Input: part model. Units: mm. Frame: model coordinates. A direction names the side the tool comes from. Coordinates: 2 decimals unless noted, no trailing zeros. Order: outer loops, then holes, each group sorted by start corner. A loop starts at its lowest first (then second) coordinate and runs counter-clockwise, first axis right, second up. Notation, with made-up numbers: (-13.75, -18) - (-7.75, -18) arc R20 ccw to (-7.75, -12) - close; hole circle Ø11 at (-39, 3.25). An arc over 180 degrees is marked (long way). Answer as CSV lines item,"result". Start each with the question number.
Item 1: First-contact query: pin 1 (8 mm diameter, centred on y = 14, z = 7.5, fed in from +X); pin 2 (8 mm diameter, centred on x = 8, z = -5, fed in from +Y); pin 3 (6 mm diameter, centred on x = -14.72, y = -8.5, fed in from +Z); pin 4 (6 mm diameter, centred on x = 0, y = -17, fed in from -Z). Flat tips, straight axial feed; report the tip coordinate or a pass-through.
Item 2: Draft query along X for faces 3 (the cylindrical face through (14.18, -10.94, 5.07)), 4 (the flat face through (4, -4, 10)), 5 (the cylindrical face through (-11.923, -3.755, -7.395)). Return one class per face: +X half, -X half, draft (parallel to the pull), parting line (faces both ways), or undercut.
Item 3: Section D-D (z = -5). Output: boundary loops of the cut face in (x, y).
Item 4: Section B-B (y = -8.5). Output: boundary loops of the cut face in (x, z).
Item 5: Section C-C (y = 0). Output: boundary loops of the cut face in (x, z), and give its area (3 significant figures).
Item 6: Access query for faces 1 (the flat face through (9, -9, 0)), 2 (the cylindrical face through (14.18, 6.06, 5.07)). Directions: +Z, -Z, +X, -X, +Y, -Y. A direction counts if a zero-diameter tool reaches every point of the face in a straight line with its end or side. Return the directions, or none.
Item 7: Section A-A (x = 0). Output: boundary loops of the cut face in (y, z), and give its area (3 significant figures).
Item 8: Material intervals for line 1 along Y through (x, z) = (0, 3.25); line 2 along X through (y, z) = (8.5, 3.5); line 3 along Y through (x, z) = (-2, 5), sorted ascending.
Autodesk Inventor part; units mm, degrees
ref_plane "YZ Plane" through (0, 0, 0) normal (1, 0, 0) x (0, 1, 0)
ref_plane "XZ Plane" through (0, 0, 0) normal (0, 1, 0) x (-1, 0, 0)
ref_plane "XY Plane" through (0, 0, 0) normal (0, 0, 1) x (1, 0, 0)
sketch "Szkic1" plane through (0, 0, 0) normal (0, 0, 1) x (1, 0, 0)
  circle A0 centre (0, 0) radius 21
  dimension "d0" = 42
extrude "Wyciągnięcie proste1" add sketch "Szkic1" along normal blind 10
sketch "Szkic2" plane through (0, 0, 10) normal (0, 0, 1) x (1, 0, 0)
  circle A0 centre (0, 0) radius 17
  circle A1 centre (0, 17) radius 2.5
  circle A2 centre (14.7224, 8.5) radius 2.5
  circle A3 centre (14.7224, -8.5) radius 2.5
  circle A4 centre (0, -17) radius 2.5
  circle A5 centre (-14.7224, -8.5) radius 2.5
  circle A6 centre (-14.7224, 8.5) radius 2.5
  dimension "d3" = 34
  dimension "d4" = 5
  dimension "d7" = 360
extrude "Wyciągnięcie proste2" cut sketch "Szkic2" against normal up to next contours A2 A0 | A0 A2 | A3 A0 | A0 A3 | A1 A0 | A0 A1 | A4 A0 | A0 A4 | A6 A0 | A0 A6 | A5 A0 | A0 A5
sketch "Szkic3" plane through (0, 0, 10) normal (0, 0, 1) x (1, 0, 0)
  circle A0 centre (0, 0) radius 5
  dimension "d11" = 10
extrude "Wyciągnięcie proste3" cut sketch "Szkic3" against normal up to next
sketch "Szkic4" plane through (0, 0, 0) normal (0, 0, -1) x (-1, 0, 0)
  circle A0 centre (0, 0) radius 5
  circle A1 centre (0, 0) radius 12.5
  dimension "d14" = 25
extrude "Wyciągnięcie proste4" add sketch "Szkic4" along normal blind 15
thread "Gwint1"
properties part number "Nakrętka trapezowa kołnierzowa JFRM-2525TR10x3"
Determined:
1,pin 1,"stops at x = 18.47"
1,pin 2,"stops at y = 11.84"
1,pin 3,"stops at z = 10"
1,pin 4,"stops at z = 0"
2,face 3,"undercut"
2,face 4,"draft"
2,face 5,"parting line"
3,outline,"circle Ø25 at (0, 0); hole circle Ø10 at (0, 0)"
4,outline,"(-19.2, 0) - (-17.22, 0) - (-17.22, 10) - (-19.2, 10) - close; (-12.22, 0) - (-9.17, 0) - (-9.17, -15) - (9.17, -15) - (9.17, 0) - (12.22, 0) - (12.22, 10) - (-12.22, 10) - close; (17.22, 0) - (19.2, 0) - (19.2, 10) - (17.22, 10) - close"
5,outline,"(-21, 0) - (-12.5, 0) - (-12.5, -15) - (-5, -15) - (-5, 10) - (-21, 10) - close; (5, -15) - (12.5, -15) - (12.5, 0) - (21, 0) - (21, 10) - (5, 10) - close"
5,area,"545 mm^2"
6,face 1,"-Z"
6,face 2,"+Z, -Z"
7,outline,"(-21, 0) - (-19.5, 0) - (-19.5, 10) - (-21, 10) - close; (-14.5, 0) - (-12.5, 0) - (-12.5, -15) - (-5, -15) - (-5, 10) - (-14.5, 10) - close; (5, -15) - (12.5, -15) - (12.5, 0) - (14.5, 0) - (14.5, 10) - (5, 10) - close; (19.5, 0) - (21, 0) - (21, 10) - (19.5, 10) - close"
7,area,"445 mm^2"
8,line 1,"y = -21 to -19.5, -14.5 to -5, 5 to 14.5, 19.5 to 21"
8,line 2,"x = -19.2 to -17.22, -12.22 to 12.22, 17.22 to 19.2"
8,line 3,"y = -20.9 to -18.5, -15.5 to -4.58, 4.58 to 15.5, 18.5 to 20.9"
